Verification items for the finished model (mm, model axes). Round coordinates to 2 decimals unless told otherwise and drop trailing zeros. Order: outer loops, then holes, each group sorted by start corner. A loop starts at its lowest first (then second) coordinate and runs counter-clockwise, first axis right, second up. Notation, with made-up numbers: M 2,77.25 L 14,77.25 A31 cw 14,109.25 Z; hole C 64.25,16.25 d3. An arc over 180 degrees is marked long. Return JSON: item names as keys, results as strings. Group by question number.
from build123d import *

# Parameters (mm, degrees)
SKETCH1_R           = 2
BOSS_EXTRUDE1_DEPTH = 3


with BuildPart() as part:
    # Sketch1 → Boss-Extrude1 (new body)
    with BuildSketch(Plane.XY):
        Polygon((18, -22.070954543), (18, 48.929045457), (-3, 48.929045457), (-3, 52.929045457), (-24, 52.929045457), (-24, 48.929045457), (-40, 48.929045457), (-40, -227.070954543), (18, -227.070954543), (18, -182.070954543), (38, -182.070954543), (38, -22.070954543), align=None)
        with Locations((28, -36.070954543)):
            Circle(SKETCH1_R, mode=Mode.SUBTRACT)
        with BuildLine():
            Line((-25.70047512, -207.785634012), (6.29952488, -207.785634012))
            ThreePointArc((6.29952488, -207.785634012), (7.006631662, -208.078527231), (7.29952488, -208.785634012))
            Line((7.29952488, -208.785634012), (7.29952488, -209.785634012))
            ThreePointArc((7.29952488, -209.785634012), (7.006631662, -210.492740793), (6.29952488, -210.785634012))
            Line((6.29952488, -210.785634012), (-25.70047512, -210.785634012))
            ThreePointArc((-25.70047512, -210.785634012), (-26.407581901, -210.492740793), (-26.70047512, -209.785634012))
            Line((-26.70047512, -209.785634012), (-26.70047512, -208.785634012))
            ThreePointArc((-26.70047512, -208.785634012), (-26.407581901, -208.078527231), (-25.70047512, -207.785634012))
        make_face(mode=Mode.SUBTRACT)
        with BuildLine():
            Line((-25.70047512, -202.785634012), (6.29952488, -202.785634012))
            ThreePointArc((6.29952488, -202.785634012), (7.006631662, -203.078527231), (7.29952488, -203.785634012))
            Line((7.29952488, -203.785634012), (7.29952488, -204.785634012))
            ThreePointArc((7.29952488, -204.785634012), (7.006631662, -205.492740793), (6.29952488, -205.785634012))
            Line((6.29952488, -205.785634012), (-25.70047512, -205.785634012))
            ThreePointArc((-25.70047512, -205.785634012), (-26.407581901, -205.492740793), (-26.70047512, -204.785634012))
            Line((-26.70047512, -204.785634012), (-26.70047512, -203.785634012))
            ThreePointArc((-26.70047512, -203.785634012), (-26.407581901, -203.078527231), (-25.70047512, -202.785634012))
        make_face(mode=Mode.SUBTRACT)
        with BuildLine():
            Line((-25.70047512, -197.785634012), (6.29952488, -197.785634012))
            ThreePointArc((6.29952488, -197.785634012), (7.006631662, -198.078527231), (7.29952488, -198.785634012))
            Line((7.29952488, -198.785634012), (7.29952488, -199.785634012))
            ThreePointArc((7.29952488, -199.785634012), (7.006631662, -200.492740793), (6.29952488, -200.785634012))
            Line((6.29952488, -200.785634012), (-25.70047512, -200.785634012))
            ThreePointArc((-25.70047512, -200.785634012), (-26.407581901, -200.492740793), (-26.70047512, -199.785634012))
            Line((-26.70047512, -199.785634012), (-26.70047512, -198.785634012))
            ThreePointArc((-26.70047512, -198.785634012), (-26.407581901, -198.078527231), (-25.70047512, -197.785634012))
        make_face(mode=Mode.SUBTRACT)
        with BuildLine():
            Line((-25.70047512, -192.785634012), (6.29952488, -192.785634012))
            ThreePointArc((6.29952488, -192.785634012), (7.006631662, -193.078527231), (7.29952488, -193.785634012))
            Line((7.29952488, -193.785634012), (7.29952488, -194.785634012))
            ThreePointArc((7.29952488, -194.785634012), (7.006631662, -195.492740793), (6.29952488, -195.785634012))
            Line((6.29952488, -195.785634012), (-25.70047512, -195.785634012))
            ThreePointArc((-25.70047512, -195.785634012), (-26.407581901, -195.492740793), (-26.70047512, -194.785634012))
            Line((-26.70047512, -194.785634012), (-26.70047512, -193.785634012))
            ThreePointArc((-26.70047512, -193.785634012), (-26.407581901, -193.078527231), (-25.70047512, -192.785634012))
        make_face(mode=Mode.SUBTRACT)
        with BuildLine():
            Line((-25.70047512, -187.785634012), (6.29952488, -187.785634012))
            ThreePointArc((6.29952488, -187.785634012), (7.006631662, -188.078527231), (7.29952488, -188.785634012))
            Line((7.29952488, -188.785634012), (7.29952488, -189.785634012))
            ThreePointArc((7.29952488, -189.785634012), (7.006631662, -190.492740793), (6.29952488, -190.785634012))
            Line((6.29952488, -190.785634012), (-25.70047512, -190.785634012))
            ThreePointArc((-25.70047512, -190.785634012), (-26.407581901, -190.492740793), (-26.70047512, -189.785634012))
            Line((-26.70047512, -189.785634012), (-26.70047512, -188.785634012))
            ThreePointArc((-26.70047512, -188.785634012), (-26.407581901, -188.078527231), (-25.70047512, -187.785634012))
        make_face(mode=Mode.SUBTRACT)
        with Locations((28, -142.070954543)):
            Circle(SKETCH1_R, mode=Mode.SUBTRACT)
    extrude(amount=BOSS_EXTRUDE1_DEPTH)


solid = part.part
1. Cross-section at B-B (y = -13.5). Enter the section's corners in (x, z), plus the area to 3 significant figures.
2. Go/stop test with flat-tipped pins: pin 1 (0.9 mm diameter, centred on y = 24.5, z = 1, fed in from +X); pin 2 (1.5 mm diameter, centred on x = -34, z = 1, fed in from +Y); pin 3 (0.9 mm diameter, centred on y = 50, z = 1.5, fed in from -X). Record where each tip stops, or that it passes through.
3. Cross-section at C-C (z = 2.2). Give the number of separate pieces and of enclosed holes in the cut face, plus the area to 3 significant figures.
4. Cross-section at A-A (x = -18.5). Enter the section's corners in (y, z), plus the area to 3 significant figures.
5. Thickness scan on line 1 along Y through (x, z) = (28, 2.25); line 2 along Y through (x, z) = (-11, 0.6); line 3 along X through (y, z) = (-209, 2.2). Record the ranges inside material, lowest first. Write a range as from..to.
Computed:
{
 "1": {"outline": "M -40,0 L 18,0 L 18,3 L -40,3 Z", "area": "174 mm²"},
 "2": {"pin 1": "stops at x = 18", "pin 2": "stops at y = 48.93", "pin 3": "stops at x = -24"},
 "3": {"separate pieces": "1", "enclosed holes": "7", "area": "18,800 mm²"},
 "4": {"outline": "M -227.07,0 L -210.79,0 L -210.79,3 L -227.07,3 Z; M -207.79,0 L -205.79,0 L -205.79,3 L -207.79,3 Z; M -202.79,0 L -200.79,0 L -200.79,3 L -202.79,3 Z; M -197.79,0 L -195.79,0 L -195.79,3 L -197.79,3 Z; M -192.79,0 L -190.79,0 L -190.79,3 L -192.79,3 Z; M -187.79,0 L 52.93,0 L 52.93,3 L -187.79,3 Z", "area": "795 mm²"},
 "5": {"line 1": "y = -182.07..-144.07, -140.07..-38.07, -34.07..-22.07", "line 2": "y = -227.07..-210.79, -207.79..-205.79, -202.79..-200.79, -197.79..-195.79, -192.79..-190.79, -187.79..52.93", "line 3": "x = -40..-26.7, 7.3..18"}
}
